The model under review builds one solid part; all positions refer to its coordinate system, in mm. A direction names the side the tool comes from. Give positions to 0.01 mm unless a question says otherwise; leave off trailing zeros. Write each loop counter-clockwise with the first axis right and the second up, starting at its lowest first coordinate (ties: lowest second). Pieces come first, ordered by that corner, then holes. Notation, with made-up numbers: (-21, 66.25) -> (38, 66.25) arc R25 cw to (38, 91.25) -> close; hole circle Ø11 at (48.25, -28.75). An arc over 180 degrees is marked (long way). Use CSV: the item, a comma, the result in double quotes.
```python
from build123d import *

# Parameters (mm, degrees)
SKETCH_1_W               = 7.5
SKETCH_1_H               = 30.5
EXTRUDE_1_DEPTH          = 3.3
SKETCH_4_W               = 7.5
SKETCH_4_H               = 8.198435562
CUT_EXTRUDE_1_DEPTH      = 17.047273912
SKETCH_2_R               = 9.25
EXTRUDE_2_DEPTH          = 15.5
SKETCH_5_R               = 4.8
CUT_EXTRUDE_2_DEPTH      = 34.218562582
CUT_EXTRUDE_3_DEPTH      = 2.75
CUT_EXTRUDE_3_DEPTH_BACK = 10
SKETCH_6_R               = 6.75
EXTRUDE_START            = -0.5
EXTRUDE_3_DEPTH          = 0.5


with BuildPart() as part:
    # 草图1 → 凸台-拉伸1 (new body)
    with BuildSketch(Plane.XY):
        Rectangle(SKETCH_1_W, SKETCH_1_H)
    extrude(amount=EXTRUDE_1_DEPTH)

    # 草图4 → 切除-拉伸1 (cut, through all)
    with BuildSketch(Plane(origin=(0, 0, 0), x_dir=(-1, 0, 0), z_dir=(0, 0, -1))):
        with Locations((0, -11.150782219)):
            Rectangle(SKETCH_4_W, SKETCH_4_H)
    extrude(amount=-CUT_EXTRUDE_1_DEPTH, mode=Mode.SUBTRACT)

    # 草图2 → 凸台-拉伸2 (add)
    with BuildSketch(Plane.XY.offset(3.3)):
        with Locations((0, -4.98)):
            Circle(SKETCH_2_R)
    extrude(amount=-EXTRUDE_2_DEPTH)

    # 草图5 → 切除-拉伸2 (cut, through all)
    with BuildSketch(Plane(origin=(0, 15.25, 0), x_dir=(1, 0, 0), z_dir=(0, 1, 0))):
        with Locations(Location((0, 4.7, 0), (0, 0, 270))):
            Circle(SKETCH_5_R)
    extrude(amount=-CUT_EXTRUDE_2_DEPTH, mode=Mode.SUBTRACT)

    # 草图6 → 切除-拉伸3 (cut, two sides: drawn at the far end of the back side and taken through both)
    with BuildSketch(Plane(origin=(0, -6, 0), x_dir=(1, 0, 0), z_dir=(0, 1, 0)).offset(-CUT_EXTRUDE_3_DEPTH_BACK)):
        with Locations(Location((0, 4.7, 0), (0, 0, 90))):
            Circle(SKETCH_6_R)
    extrude(amount=CUT_EXTRUDE_3_DEPTH + CUT_EXTRUDE_3_DEPTH_BACK, mode=Mode.SUBTRACT)

    # 草图7 → 凸台-拉伸3 (add)
    with BuildSketch(Plane(origin=(0, 0, 0), x_dir=(-1, 0, 0), z_dir=(0, 0, -1)).offset(EXTRUDE_START)):
        with BuildLine():
            Line((-0.974679434, 15.25), (-0.974679434, 4.218505313))
            ThreePointArc((-0.974679434, 4.218505313), (0, 4.27), (0.974679434, 4.218505313))
            Line((0.974679434, 4.218505313), (0.974679434, 15.25))
            Line((0.974679434, 15.25), (-0.974679434, 15.25))
        make_face()
    extrude(amount=EXTRUDE_3_DEPTH)


solid = part.part
```
Q1. Machinability: for faces 4 (the flat face through (3.75, 9, 2)), 5 (the flat face through (-3.75, 9, 2)), 6 (the cylindrical face through (2.585, -7.604, -10.935)), which of the approach directions +Z, -Z, +X, -X, +Y, -Y give a long, thin tool a straight path to every point of the face, cutting with its end or side? Answer none if there is none.
Derived:
face 4,"+Z, -Z, +X, +Y"
face 5,"+Z, -Z, -X, +Y"
face 6,"-Y"
Q2. Consider section B-B (z = -0.75). Write out the cut boundary in (x, y).
Derived:
outline,"(-5.47, -12.44) -> (-5.47, -3.25) -> (-2.73, -3.25) -> (-2.73, 3.86) arc R9.25 ccw to start; (2.73, -3.25) -> (5.47, -3.25) -> (5.47, -12.44) arc R9.25 ccw to (2.73, 3.86) -> close"
Q3. Consider section C-C (y = -4.98). Write out the cut boundary in (x, z).
Derived:
outline,"(-9.25, -12.2) -> (9.25, -12.2) -> (9.25, 3.3) -> (-9.25, 3.3) -> close; hole circle Ø13.5 at (0, -4.7)"
Q4. The part is to be moulded in two halves that separate along X. For faces 1 (the cylindrical face through (5, 2.8, -4.3)), 2 (the cylindrical face through (1.44, 0.57, -0.12)), 3 (the flat face through (0, -5, -12.2)), say which applies: pulls with the +X half, pulls with the -X half, needs draft (parallel to the pull), parting line crosses it, or undercut.
Derived:
face 1,"parting line crosses it"
face 2,"undercut"
face 3,"needs draft"
Q5. Consider section A-A (x = 0). Write out the cut boundary in (y, z).
Derived:
outline,"(-14.23, -12.2) -> (4.27, -12.2) -> (4.27, -9.5) -> (-3.25, -9.5) -> (-3.25, -11.45) -> (-14.23, -11.45) -> close; (-14.23, 2.05) -> (-3.25, 2.05) -> (-3.25, 0.1) -> (4.27, 0.1) -> (4.27, 0) -> (15.25, 0) -> (15.25, 3.3) -> (-14.23, 3.3) -> close"
Q6. To check wall thickness, follow probe 1 along Z at (x, y) = (0, -1.5); probe 2 along Z at (x, y) = (3, -11.75); probe 3 along X at (y, z) = (-6.5, -3). State the ranges of each line that lie inside material, in increasing order.
Derived:
probe 1,"z = -12.2 to -9.5, 0.1 to 3.3"
probe 2,"z = -12.2 to -10.75, 1.35 to 3.3"
probe 3,"x = -9.12 to -6.53, 6.53 to 9.12"
Q7. Insertion check: pin 1 (2.5 mm diameter, centred on y = 12, z = 1, fed in from +X); pin 2 (6 mm diameter, centred on x = -3.5, z = -6, fed in from +Y); pin 3 (4 mm diameter, centred on x = 5.5, z = -8, fed in from +Y); pin 4 (6 mm diameter, centred on y = -4.5, z = -1, fed in from -X). Each pin has a flat end and moves straight along its axis. Give the tip position at first contact, or say it passes through.
Derived:
pin 1,"stops at x = 3.75"
pin 2,"stops at y = 3.93"
pin 3,"stops at y = 3.58"
pin 4,"stops at x = -9.25"
Q8. Consider section D-D (x = -2.5). Write out the cut boundary in (y, z), then the cut area to 3 significant figures.
Derived:
outline,"(-13.89, -12.2) -> (3.93, -12.2) -> (3.93, -8.8) -> (-3.25, -8.8) -> (-3.25, -10.97) -> (-13.89, -10.97) -> close; (-13.89, 1.57) -> (-3.25, 1.57) -> (-3.25, -0.6) -> (3.93, -0.6) -> (3.93, 0) -> (15.25, 0) -> (15.25, 3.3) -> (-13.89, 3.3) -> close"
area,"121 mm2"
